Verification items for the finished model (mm, model axes). A direction names the side the tool comes from. Round coordinates to 2 decimals unless told otherwise and drop trailing zeros. Order: outer loops, then holes, each group sorted by start corner. A loop starts at its lowest first (then second) coordinate and runs counter-clockwise, first axis right, second up. Notation, with made-up numbers: M 59,-30 L 90,-30 A27 ccw 90,-12 Z; hole C 24,16 d8. An arc over 180 degrees is marked long. Return JSON: item names as keys, results as strings. Group by question number.
from build123d import *

# Parameters (mm, degrees)
ESQUISSE1_W                  = 6.94
ESQUISSE1_H                  = 12.9
BOSS_EXTRU_1_DEPTH           = 9.06
ESQUISSE2_R                  = 2.85
BOSS_EXTRU_2_DEPTH           = 8.7
ESQUISSE3_R                  = 2
ENL_V_MAT_EXTRU_1_DEPTH      = 8.7
ENL_V_START                  = -3.45
ESQUISSE4_R                  = 0.5
ENL_V_MAT_EXTRU_2_DEPTH      = 2.5
ENL_V_MAT_EXTRU_2_DEPTH_BACK = 2.5
CHANFREIN1_SIZE              = 0.25
CHANFREIN1_SIZE2             = 2.378591114
ESQUISSE5_W                  = 2.16
ESQUISSE5_H                  = 0.8
BOSS_EXTRU_3_DEPTH           = 4
CONG_1_R                     = 0.3
ESQUISSE6_W                  = 1.1
ESQUISSE6_H                  = 1.9
ENL_V_MAT_EXTRU_3_DEPTH      = 12.7
SCALE1_SCALE                 = 0.64015


with BuildPart() as part:
    # Esquisse1 → Boss.-Extru.1 (new body)
    with BuildSketch(Plane(origin=(0, 0, 0), x_dir=(1, 0, 0), z_dir=(0, 1, 0))):
        with Locations((3.47, 6.45)):
            Rectangle(ESQUISSE1_W, ESQUISSE1_H)
    extrude(amount=BOSS_EXTRU_1_DEPTH)

    # Esquisse2 → Boss.-Extru.2 (add)
    with BuildSketch(Plane(origin=(0, 9.06, 0), x_dir=(1, 0, 0), z_dir=(0, 1, 0))):
        with Locations((3.47, 6.45)):
            Circle(ESQUISSE2_R)
    extrude(amount=BOSS_EXTRU_2_DEPTH)

    # Esquisse3 → Enlèv. mat.-Extru.1 (cut)
    with BuildSketch(Plane(origin=(0, 17.76, 0), x_dir=(1, 0, 0), z_dir=(0, 1, 0))):
        with Locations((3.47, 6.45)):
            Circle(ESQUISSE3_R)
    extrude(amount=-ENL_V_MAT_EXTRU_1_DEPTH, mode=Mode.SUBTRACT)

    # Esquisse4 → Enlèv. mat.-Extru.2 (cut, two sides)
    with BuildSketch(Plane.ZY.offset(ENL_V_START)) as enl_v_mat_extru_2_sk:
        with Locations((-6.453279692, 14.76)):
            Circle(ESQUISSE4_R)
    extrude(amount=ENL_V_MAT_EXTRU_2_DEPTH, mode=Mode.SUBTRACT)
    extrude(enl_v_mat_extru_2_sk.sketch, amount=-ENL_V_MAT_EXTRU_2_DEPTH_BACK, mode=Mode.SUBTRACT)

    # Chanfrein1
    chanfrein1_edges = [part.edges().sort_by_distance(p)[0] for p in [
        (1.47, 17.76, -6.45),
    ]]
    chanfrein1_side = [part.faces().sort_by_distance(p)[0] for p in [
        (0.700610173, 17.76, -6.45),
    ]]
    chamfer(chanfrein1_edges, length=CHANFREIN1_SIZE, length2=CHANFREIN1_SIZE2, reference=chanfrein1_side[0])

    # Esquisse5 → Boss.-Extru.3 (add)
    with BuildSketch(Plane.XZ):
        with Locations((3.47, -1.6)):
            Rectangle(ESQUISSE5_W, ESQUISSE5_H)
        with Locations((3.47, -11.3)):
            Rectangle(ESQUISSE5_W, ESQUISSE5_H)
        with Locations((3.47, -6.45)):
            Rectangle(ESQUISSE5_W, ESQUISSE5_H)
    extrude(amount=BOSS_EXTRU_3_DEPTH)

    # Congé1
    cong_1_edges = [part.edges().sort_by_distance(p)[0] for p in [
        (2.39, -4, -1.6),
        (4.55, -4, -1.6),
        (4.55, -4, -11.3),
        (2.39, -4, -11.3),
        (2.39, -4, -6.45),
        (4.55, -4, -6.45),
    ]]
    fillet(cong_1_edges, radius=CONG_1_R)

    # Esquisse6 → Enlèv. mat.-Extru.3 (cut, through all)
    with BuildSketch(Plane(origin=(0, 0, -11.7), x_dir=(-1, 0, 0), z_dir=(0, 0, -1))):
        with Locations((-3.470290463, -2.41)):
            Rectangle(ESQUISSE6_W, ESQUISSE6_H)
    extrude(amount=-ENL_V_MAT_EXTRU_3_DEPTH, mode=Mode.SUBTRACT)


with BuildPart() as part_1:
    # Scale1: scaled about (3.47008246, 5.432983417, -6.449996817)
    add(part.part.scale(SCALE1_SCALE).moved(Location((1.248709173, 1.955059083, -2.321031355))))


solid = part_1.part
1. Thickness scan on line 1 along Z through (x, y) = (3, 0); line 2 along Y through (x, z) = (3.4, -5.75); line 3 along Z through (x, y) = (2.8, 9.5). Record the ranges inside material, lowest first. Write a range as from..to.
2. Draft check along Z on faces 4 (the face through (3, 5, -2.321)), 5 (the face through (3, 1.955, -7)), 6 (the face through (3.5, 1.3, -9.811)). Enter one of: +Z half, -Z half, draft (parallel to the pull), parting line (faces both ways), or undercut.
3. Cross-section at C-C (x = 3.35). Give the number of separate pieces and of enclosed holes in the cut face, plus the area to 3 significant figures.
4. Cross-section at B-B (y = 10.75). Enter the section's corners in (x, z).
5. Access from +Z, -Z, +X, -X, +Y, -Y to the whole of each face (thin tool, end or side, straight path). Record for faces 1 (the face through (4.7, 9.8, -6.8)), 2 (the face through (3.5, 1.3, -3.089)), 3 (the face through (3.5, 1.3, -3.601)).
6. Go/stop test with flat-tipped pins: pin 1 (0.6 mm diameter, centred on y = 0.5, z = -6.5, fed in from +X); pin 2 (1.3 mm diameter, centred on x = 3.5, z = -6, fed in from +Y); pin 3 (0.7 mm diameter, centred on x = 3, y = 1, fed in from +Z). Record where each tip stops, or that it passes through.
7. Cross-section at A-A (y = 0.75). Enter the section's corners in (x, z).
Computed:
{
 "1": {"line 1": "z = -9.81..-9.3, -6.71..-6.19, -3.6..-3.09", "line 2": "y = 1.96..7.75", "line 3": "z = -8.15..-7.54, -5.36..-4.75"},
 "2": {"face 4": "+Z half", "face 5": "undercut", "face 6": "-Z half"},
 "3": {"separate pieces": "4", "enclosed holes": "0", "area": "55.8 mm²"},
 "4": {"outline": "C 3.47,-6.45 d3.65; hole C 3.47,-6.45 d2.56"},
 "5": {"face 1": "+Y", "face 2": "+Z, +X, -X, -Y", "face 3": "+X, -X, -Y"},
 "6": {"pin 1": "stops at x = 4.16", "pin 2": "stops at y = 7.75", "pin 3": "stops at z = -3.09"},
 "7": {"outline": "M 2.78,-9.81 L 3.12,-9.81 L 3.12,-9.3 L 2.78,-9.3 Z; M 2.78,-6.71 L 3.12,-6.71 L 3.12,-6.19 L 2.78,-6.19 Z; M 2.78,-3.6 L 3.12,-3.6 L 3.12,-3.09 L 2.78,-3.09 Z; M 3.82,-9.81 L 4.16,-9.81 L 4.16,-9.3 L 3.82,-9.3 Z; M 3.82,-6.71 L 4.16,-6.71 L 4.16,-6.19 L 3.82,-6.19 Z; M 3.82,-3.6 L 4.16,-3.6 L 4.16,-3.09 L 3.82,-3.09 Z"}
}
